Can you work these out from the model? Positions are in its coordinate system, mm. A direction names the side the tool comes from. Coordinates: 2 decimals unless noted, no trailing zeros. Write each loop counter-clockwise with the first axis right and the second up, starting at its lowest first coordinate (ties: lowest second). Pieces come first, ordered by that corner, then holes. Notation, with made-up numbers: (-14, -22.75) -> (17, -22.75) arc R24 ccw to (17, -11.75) -> close; hole circle Ø3 at (72, -9). An arc over 180 degrees is marked (long way). Use one line per item in the form item = value.
```python
from build123d import *

# Parameters (mm, degrees)
SKETCH1_W           = 280
SKETCH1_H           = 280
BOSS_EXTRUDE1_DEPTH = 63
SKETCH2_W           = 264
SKETCH2_H           = 264
CUT_EXTRUDE1_DEPTH  = 55
SKETCH4_R           = 15
CUT_EXTRUDE2_DEPTH  = 55


with BuildPart() as part:
    # Sketch1 → Boss-Extrude1 (new body)
    with BuildSketch(Plane(origin=(0, 0, 0), x_dir=(0, 0, -1), z_dir=(1, 0, 0))):
        Rectangle(SKETCH1_W, SKETCH1_H)
    extrude(amount=BOSS_EXTRUDE1_DEPTH)

    # Sketch2 → Cut-Extrude1 (cut)
    with BuildSketch(Plane(origin=(63, 0, 0), x_dir=(0, 0, -1), z_dir=(1, 0, 0))):
        Rectangle(SKETCH2_W, SKETCH2_H)
    extrude(amount=-CUT_EXTRUDE1_DEPTH, mode=Mode.SUBTRACT)

    # Sketch4 → Cut-Extrude2 (cut)
    with BuildSketch(Plane(origin=(8, 0, 0), x_dir=(0, 0, -1), z_dir=(1, 0, 0))):
        with Locations((107, 107)):
            Circle(SKETCH4_R)
    extrude(amount=-CUT_EXTRUDE2_DEPTH, mode=Mode.SUBTRACT)


solid = part.part
```
Q1. Suppose I cut it at D-D (y = 2.5). Write out the boundary of the cut face in (x, z), then the cut area to 3 significant figures.
Return value:
outline = (0, -140) -> (63, -140) -> (63, -132) -> (8, -132) -> (8, 132) -> (63, 132) -> (63, 140) -> (0, 140) -> close
area = 3,120 mm2
Q2. Thinking about a two-plate mould opening in Z: for faces 3 (the flat face through (36, -2, 132)), 4 (the flat face through (31, 140, 2)), 5 (the flat face through (31, -2, 140)), 6 (the flat face through (31, -2, -140)), which applies, released by +Z, released by -Z, zero draft, split by the parting line, or undercut?
Return value:
face_3 = undercut
face_4 = zero draft
face_5 = released by +Z
face_6 = released by -Z
Q3. For faces 1 (the flat face through (0, 2, 2)), 2 (the flat face through (36, 132, 2)), which set-ups out of +Z, -Z, +X, -X, +Y, -Y let a thin tool reach every point of the face, with its end or its side?
Return value:
face_1 = +Z, -Z, -X, +Y, -Y
face_2 = +X
Q4. Will this pin go through, and if not, where does the flat tip stop? pin 1 (6 mm diameter, centred on y = -81, z = 2.5, fed in from +X).
Return value:
pin_1 = 8
Q5. Suppose I cut it at C-C (x = 19.5). Write out the boundary of the cut face in (y, z), then the cut area to 3 significant figures.
Return value:
outline = (-140, -140) -> (140, -140) -> (140, 140) -> (-140, 140) -> close; hole (-132, -132) -> (132, -132) -> (132, 132) -> (-132, 132) -> close
area = 8,700 mm2
Q6. Suppose I cut it at A-A (y = 107). Write out the boundary of the cut face in (x, z), then the cut area to 3 significant figures.
Return value:
outline = (0, -140) -> (63, -140) -> (63, -132) -> (8, -132) -> (8, -122) -> (0, -122) -> close; (0, -92) -> (8, -92) -> (8, 132) -> (63, 132) -> (63, 140) -> (0, 140) -> close
area = 2,880 mm2
Q7. Suppose I cut it at B-B (z = -107). Write out the boundary of the cut face in (x, y).
Return value:
outline = (0, -140) -> (63, -140) -> (63, -132) -> (8, -132) -> (8, 92) -> (0, 92) -> close; (0, 122) -> (8, 122) -> (8, 132) -> (63, 132) -> (63, 140) -> (0, 140) -> close
Q8. If I drill on line 1 (Y direction, x = 14.5, z = 68.5); line 2 (Y direction, x = 5, z = -107), over which ranges is the centre line in solid material (lowest first)? Write a range as from..to.
Return value:
line_1 = -140..-132, 132..140
line_2 = -140..92, 122..140
